from build123d import *

# Parameters (mm, degrees)
F0_W     = 200
F0_H     = 20
F1_DEPTH = 6.35


# Not quite as in the source:
# - a length typed as a fraction of an inch, garbled in the dataset ("3 / 203.2 mm" for 3/8 in), is restored


with BuildPart() as f1:
    # F0 (on Top) → F1 (new body)
    with BuildSketch(Plane.XY):
        Rectangle(F0_W, F0_H)
        with BuildLine():
            Line((-80, 3.25), (-40, 3.25))
            ThreePointArc((-40, 3.25), (-36.75, 0), (-40, -3.25))
            Line((-40, -3.25), (-80, -3.25))
            ThreePointArc((-80, -3.25), (-83.25, 0), (-80, 3.25))
        make_face(mode=Mode.SUBTRACT)
        with BuildLine():
            Line((-20, 3.25), (20, 3.25))
            ThreePointArc((20, 3.25), (23.25, 0), (20, -3.25))
            Line((20, -3.25), (-20, -3.25))
            ThreePointArc((-20, -3.25), (-23.25, 0), (-20, 3.25))
        make_face(mode=Mode.SUBTRACT)
        with BuildLine():
            Line((80, -3.25), (40, -3.25))
            ThreePointArc((40, -3.25), (36.75, 0), (40, 3.25))
            Line((40, 3.25), (80, 3.25))
            ThreePointArc((80, 3.25), (83.25, 0), (80, -3.25))
        make_face(mode=Mode.SUBTRACT)
    extrude(amount=F1_DEPTH)


solid = f1.part
Design review of the part built by this model. Coordinates are the model's own, in mm. A direction names the side the tool comes from. Round coordinates to 2 decimals unless told otherwise and drop trailing zeros. Order: outer loops, then holes, each group sorted by start corner. A loop starts at its lowest first (then second) coordinate and runs counter-clockwise, first axis right, second up.
1) Consider section C-C (x = 78). State the section outline as (y, z) points, plus the area to 3 significant figures.
The answers:
outline: (-10, 0) - (-3.25, 0) - (-3.25, 6.35) - (-10, 6.35) - close; (3.25, 0) - (10, 0) - (10, 6.35) - (3.25, 6.35) - close
area: 85.7 mm2
2) Draft analysis for pull direction Y (two halves, no side actions). For faces 3 (the flat face through (-1, 5, 6.35)), 4 (the flat face through (60, -3.25, 3)), 5 (the flat face through (-1, -10, 3)), 6 (the flat face through (-1, 10, 3)), state which applies: released by +Y, released by -Y, zero draft, split by the parting line, or undercut.
The answers:
face 3: zero draft
face 4: undercut
face 5: released by -Y
face 6: released by +Y
3) Machinability: for faces 1 (the flat face through (-100, 0, 3)), 2 (the flat face through (0, 3.25, 3)), which of the approach directions +Z, -Z, +X, -X, +Y, -Y give a long, thin tool a straight path to every point of the face, cutting with its end or side? Answer none if there is none.
The answers:
face 1: +Z, -Z, -X, +Y, -Y
face 2: +Z, -Z
4) Consider section B-B (z = 3.5). State the section outline as (x, y) points, plus the area to 3 significant figures.
The answers:
outline: (-100, -10) - (100, -10) - (100, 10) - (-100, 10) - close; hole (-80, -3.25) - (-40, -3.25) arc R3.25 ccw to (-40, 3.25) - (-80, 3.25) arc R3.25 ccw to start; hole (-20, -3.25) - (20, -3.25) arc R3.25 ccw to (20, 3.25) - (-20, 3.25) arc R3.25 ccw to start; hole (40, -3.25) - (80, -3.25) arc R3.25 ccw to (80, 3.25) - (40, 3.25) arc R3.25 ccw to start
area: 3,120 mm2
5) Consider section A-A (y = 0). State the section outline as (x, z) points, plus the area to 3 significant figures.
The answers:
outline: (-100, 0) - (-83.25, 0) - (-83.25, 6.35) - (-100, 6.35) - close; (-36.75, 0) - (-23.25, 0) - (-23.25, 6.35) - (-36.75, 6.35) - close; (23.25, 0) - (36.75, 0) - (36.75, 6.35) - (23.25, 6.35) - close; (83.25, 0) - (100, 0) - (100, 6.35) - (83.25, 6.35) - close
area: 384 mm2
6) For L1, parallel to X at y = -0.5, z = 1; L2, parallel to Y at x = -68, z = 4.5; L3, parallel to X at y = -1.75, z = 3, list the stretches that pass through material, from the lowest coordinate up.
The answers:
L1: x = -100 to -83.21, -36.79 to -23.21, 23.21 to 36.79, 83.21 to 100
L2: y = -10 to -3.25, 3.25 to 10
L3: x = -100 to -82.74, -37.26 to -22.74, 22.74 to 37.26, 82.74 to 100
